Geometry: final body of the model. Coordinates: model frame, mm. Round coordinates to 2 decimals unless told otherwise and drop trailing zeros. Order: outer loops, then holes, each group sorted by start corner. A loop starts at its lowest first (then second) coordinate and runs counter-clockwise, first axis right, second up. Notation, with made-up numbers: (-37, -32.75) - (5, -32.75) arc R23 ccw to (5, -12.75) - close; hole circle Ø10 at (-40, -20.75). An arc over 180 degrees is marked (long way). Put each result on its own line as item: value. Start each with the question number.
(1) Pull-direction query (X, two-part tool) for faces 1 (the face through (-1, 1, 3.175)), 2 (the face through (-21.205, 4, 2)), 3 (the face through (42.397, 13.352, 1.565)); classes: released by +X, released by -X, zero draft, split by the parting line, or undercut.
(2) Section B-B (y = 31.75). Output: boundary loops of the cut face in (x, z) (3 decimals), and give its area (3 significant figures).
(3) Material intervals for L1, parallel to Y at x = 27.5, z = 2.45; L2, parallel to X at y = 11.5, z = 2.65; L3, parallel to Y at x = -24.5, z = 2.25, sorted ascending. Write a range as [from, to].
(4) Section C-C (z = 1.2). Count the separate pieces of the cut face and the enclosed holes in it, and give its area (3 significant figures).
(5) Section A-A (x = 0). Output: boundary loops of the cut face in (y, z) (3 decimals), and give its area (3 significant figures).
(6) Pin query (flat end, axial travel): P1, Ø1, axis at x = 26, z = 1.5, coming from the +Y side; P2, Ø1, axis at y = 4.5, z = 1.5, coming from the +X side; P3, Ø1, axis at y = 5.5, z = 1.5, coming from the -X side. Return the tip coordinate at first contact, or that it passes through.
from build123d import *

# Parameters (mm, degrees)
F0_R     = 44.45
F0_R_2   = 6.35
F1_DEPTH = 3.175


with BuildPart() as f1:
    # F0 (on Top) → F1 (new body)
    with BuildSketch(Plane.XY):
        Circle(F0_R)
        with BuildLine():
            Line((-21.2053465663, 12.6017319805), (-18.0090443844, 12.6017319805))
            Line((-18.0090443844, 12.6017319805), (-18.0090443844, -5.1916187724))
            add(Edge.make_bspline(
                [(-18.0090443844, -5.1916187724), (-18.0090443844, -9.8987907239), (-20.8502018794, -12.5894631821)],
                knots=[0, 0, 0, 1, 1, 1], degree=2))
            add(Edge.make_bspline(
                [(-20.8502018794, -12.5894631821), (-23.6913593745, -15.2801356403), (-28.6573655893, -15.2801356403)],
                knots=[0, 0, 0, 1, 1, 1], degree=2))
            add(Edge.make_bspline(
                [(-28.6573655893, -15.2801356403), (-33.6233718042, -15.2801356403), (-36.341131569, -12.568395277)],
                knots=[0, 0, 0, 1, 1, 1], degree=2))
            add(Edge.make_bspline(
                [(-36.341131569, -12.568395277), (-39.0588913339, -9.8566549136), (-39.0588913339, -5.1193859547)],
                knots=[0, 0, 0, 1, 1, 1], degree=2))
            Line((-39.0588913339, -5.1193859547), (-39.0588913339, 12.6017319805))
            Line((-39.0588913339, 12.6017319805), (-35.8565697505, 12.6017319805))
            Line((-35.8565697505, 12.6017319805), (-35.8565697505, -5.3421038092))
            add(Edge.make_bspline(
                [(-35.8565697505, -5.3421038092), (-35.8565697505, -8.7852014515), (-33.9755067903, -10.6301480028)],
                knots=[0, 0, 0, 1, 1, 1], degree=2))
            add(Edge.make_bspline(
                [(-33.9755067903, -10.6301480028), (-32.0944438301, -12.4750945541), (-28.4466865378, -12.4750945541)],
                knots=[0, 0, 0, 1, 1, 1], degree=2))
            add(Edge.make_bspline(
                [(-28.4466865378, -12.4750945541), (-24.9674724866, -12.4750945541), (-23.0864095265, -10.6211189006)],
                knots=[0, 0, 0, 1, 1, 1], degree=2))
            add(Edge.make_bspline(
                [(-23.0864095265, -10.6211189006), (-21.2053465663, -8.7671432471), (-21.2053465663, -5.3059874003)],
                knots=[0, 0, 0, 1, 1, 1], degree=2))
            Line((-21.2053465663, -5.3059874003), (-21.2053465663, 12.6017319805))
        make_face(mode=Mode.SUBTRACT)
        with BuildLine():
            Line((4.0159456036, -14.9009133476), (1.4396417734, -14.9009133476))
            Line((1.4396417734, -14.9009133476), (-7.890430509, 9.4776626162))
            Line((-7.890430509, 9.4776626162), (-8.0409155459, 9.4776626162))
            add(Edge.make_bspline(
                [(-8.0409155459, 9.4776626162), (-7.7760618811, 6.5823305079), (-7.7760618811, 2.5914673316)],
                knots=[0, 0, 0, 1, 1, 1], degree=2))
            Line((-7.7760618811, 2.5914673316), (-7.7760618811, -14.9009133476))
            Line((-7.7760618811, -14.9009133476), (-10.7315880041, -14.9009133476))
            Line((-10.7315880041, -14.9009133476), (-10.7315880041, 12.6017319805))
            Line((-10.7315880041, 12.6017319805), (-5.916066826, 12.6017319805))
            Line((-5.916066826, 12.6017319805), (2.7940071047, -10.0853921695))
            Line((2.7940071047, -10.0853921695), (2.9444921415, -10.0853921695))
            Line((2.9444921415, -10.0853921695), (11.72679889, 12.6017319805))
            Line((11.72679889, 12.6017319805), (16.5062036592, 12.6017319805))
            Line((16.5062036592, 12.6017319805), (16.5062036592, -14.9009133476))
            Line((16.5062036592, -14.9009133476), (13.3099014773, -14.9009133476))
            Line((13.3099014773, -14.9009133476), (13.3099014773, 2.8202045876))
            add(Edge.make_bspline(
                [(13.3099014773, 2.8202045876), (13.3099014773, 5.8660217327), (13.574755142, 9.4415462074)],
                knots=[0, 0, 0, 1, 1, 1], degree=2))
            Line((13.574755142, 9.4415462074), (13.4242701052, 9.4415462074))
            Line((13.4242701052, 9.4415462074), (4.0159456036, -14.9009133476))
        make_face(mode=Mode.SUBTRACT)
        Polygon((27.2448158862, -3.1450222717), (27.2448158862, -14.9009133476), (24.0485137043, -14.9009133476), (24.0485137043, 12.6017319805), (39.3799292548, 12.6017319805), (39.3799292548, 9.7605744854), (27.2448158862, 9.7605744854), (27.2448158862, -0.3038647767), (38.6455622752, -0.3038647767), (38.6455622752, -3.1450222717), align=None, mode=Mode.SUBTRACT)
        with Locations((0, 31.75)):
            Circle(F0_R_2, mode=Mode.SUBTRACT)
    extrude(amount=F1_DEPTH)


solid = f1.part
Checks:
1. face 1: zero draft
1. face 2: undercut
1. face 3: split by the parting line
2. outline: (-31.109, 0) - (-6.35, 0) - (-6.35, 3.175) - (-31.109, 3.175) - close; (6.35, 0) - (31.109, 0) - (31.109, 3.175) - (6.35, 3.175) - close
2. area: 157 mm²
3. L1: y = [-34.92, -3.15], [-0.3, 9.76], [12.6, 34.92]
3. L2: x = [-42.94, -39.06], [-35.86, -21.21], [-18.01, -10.73], [-5.49, 11.3], [16.51, 24.05], [39.38, 42.94]
3. L3: y = [-37.09, -14.7], [-11.64, 37.09]
4. separate pieces: 1
4. enclosed holes: 4
4. area: 5,400 mm²
5. outline: (-44.45, 0) - (-11.139, 0) - (-11.139, 3.175) - (-44.45, 3.175) - close; (-2.808, 0) - (25.4, 0) - (25.4, 3.175) - (-2.808, 3.175) - close; (38.1, 0) - (44.45, 0) - (44.45, 3.175) - (38.1, 3.175) - close
5. area: 215 mm²
6. P1: stops at y = 36.41
6. P2: stops at x = 44.27
6. P3: stops at x = -44.17
